Geometry: see drawing. Coordinates: mm, zero at the bounding-box minimum. A direction names the side the tool comes from. Coordinates: 2 decimals unless noted, no trailing zeros. Order: outer loops, then holes, each group sorted by start corner. A loop starts at its lowest first (then second) coordinate and runs counter-clockwise, first axis right, second up.
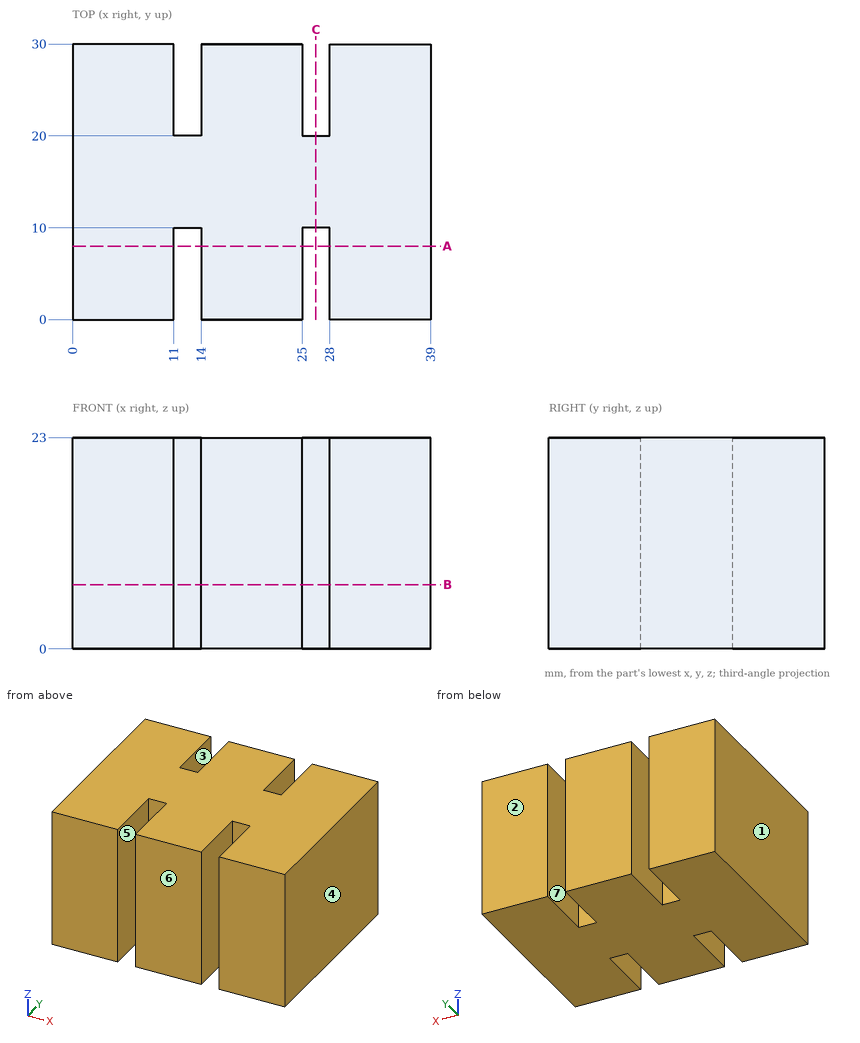
Q1. Material intervals for line 1 along X through (y, z) = (2.5, 11.75); line 2 along Y through (x, z) = (27, 20.5), sorted ascending.
Solutions:
line 1: x = 0 to 11, 14 to 25, 28 to 39
line 2: y = 10 to 20
Q2. Set-up query: the marked faces 5, 6 and 7. Return all of +Z, -Z, +X, -X, +Y, -Y with unobstructed straight access to the full face (end or side cutting, diameter ignored); none if empty.
Solutions:
face 5: +Z, -Z, -Y
face 6: +Z, -Z, +X, -X, -Y
face 7: +Z, -Z, +Y
Q3. Pull-direction query (X, two-part tool) for the marked faces 1, 2, 3 and 4; classes: pulls with the +X half, pulls with the -X half, needs draft (parallel to the pull), parting line crosses it, or undercut.
Solutions:
face 1: pulls with the -X half
face 2: needs draft
face 3: undercut
face 4: pulls with the +X half
Q4. Section query B-B on z = 7. Output: boundary loops of the cut face in (x, y).
Solutions:
outline: (0, 0) - (11, 0) - (11, 10) - (14, 10) - (14, 0) - (25, 0) - (25, 10) - (28, 10) - (28, 0) - (39, 0) - (39, 30) - (28, 30) - (28, 20) - (25, 20) - (25, 30) - (14, 30) - (14, 20) - (11, 20) - (11, 30) - (0, 30) - close
Q5. Section query C-C on x = 26.5. Output: boundary loops of the cut face in (y, z).
Solutions:
outline: (10, 0) - (20, 0) - (20, 23) - (10, 23) - close
Q6. Section query A-A on y = 8. Output: boundary loops of the cut face in (x, z), plus the area to 3 significant figures.
Solutions:
outline: (0, 0) - (11, 0) - (11, 23) - (0, 23) - close; (14, 0) - (25, 0) - (25, 23) - (14, 23) - close; (28, 0) - (39, 0) - (39, 23) - (28, 23) - close
area: 759 mm2
Q7. Pin query (flat end, axial travel): P1, Ø0.9, axis at x = 26, z = 15, coming from the -Y side; P2, Ø2.5, axis at x = 26.5, z = 9, coming from the +Y side. Return the tip coordinate at first contact, or that it passes through.
Solutions:
P1: stops at y = 10
P2: stops at y = 20
